Can you work these out from the model? Positions are in its coordinate system, mm. Face numbers are marked on the shaded views. A direction names the side the tool comes from. Coordinates: 2 decimals unless noted, no trailing zeros. Order: outer loops, then holes, each group sorted by start corner. A loop starts at its lowest first (then second) coordinate and runs counter-clockwise, first axis right, second up. Notation, with made-up numbers: (-40, 25.25) -> (16, 25.25) arc R15 cw to (16, 31.25) -> close; hole circle Ø5 at (1.25, 75.25). An arc over 180 degrees is marked (long way). Use a Markdown table: item, result. Add a question column.
1. Suppose I cut it at A-A, the plane x = 0. List the corners of the cut face in (y, z) for me, then the cut area to 3 significant figures.
2. Suppose I cut it at C-C, the plane z = 22. List the corners of the cut face in (x, y) for me, then the cut area to 3 significant figures.
3. Suppose I cut it at B-B, the plane z = 0. List the corners of the cut face in (x, y) for me, then the cut area to 3 significant figures.
4. If I drill on line 1 along Z through (x, y) = (0, -9.4); line 2 along Z through (x, y) = (0, -4.25); line 3 along Y through (x, z) = (-7, 26), over which ranges is the centre line in solid material (lowest first)? Write a range as from..to.
5. Suppose I cut it at D-D, the plane y = -4.75. List the corners of the cut face in (x, z) for me, then the cut area to 3 significant figures.
6. For pin 1 Ø3 at (y, z) = (-3.5, -15.5) entering from -X; pin 2 Ø1.5 at (y, z) = (-3.5, 8.5) entering from +X; pin 3 Ø5 at (x, y) = (-15.5, -1.5) entering from +Z, each with a flat end and sliding along its axis, tell me the tip position at first contact or that it passes through.
7. For the marked faces 1 and 2, which set-ups out of +Z, -Z, +X, -X, +Y, -Y let a thin tool reach every point of the face, with its end or its side?
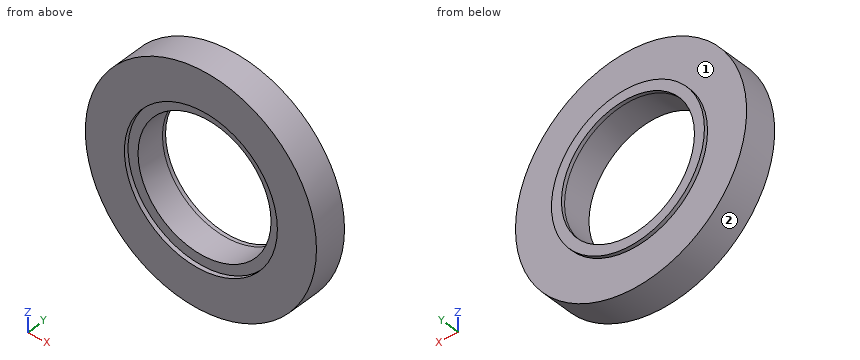
```python
from build123d import *

# Parameters (mm, degrees)
F0_R     = 34.75
F0_R_2   = 20
F1_DEPTH = 10
F2_R     = 23
F2_R_2   = 20
F3_DEPTH = 1.3
F4_R     = 23
F4_R_2   = 20
F5_DEPTH = 1.1


with BuildPart() as f1:
    # F0 (on Front) → F1 (new body)
    with BuildSketch(Plane.XZ):
        Circle(F0_R)
        Circle(F0_R_2, mode=Mode.SUBTRACT)
    extrude(amount=F1_DEPTH)

    # F2 (on face) → F3 (cut)
    with BuildSketch(Plane.XZ.offset(10)):
        Circle(F2_R)
        Circle(F2_R_2, mode=Mode.SUBTRACT)
    extrude(amount=-F3_DEPTH, mode=Mode.SUBTRACT)

    # F4 (on face) → F5 (join)
    with BuildSketch(Plane(origin=(0, 0, 0), x_dir=(-1, 0, 0), z_dir=(0, 1, 0))):
        Circle(F4_R)
        Circle(F4_R_2, mode=Mode.SUBTRACT)
    extrude(amount=F5_DEPTH)


solid = f1.part
```
Worked out:
| question | item | result |
|---|---|---|
| 1 | outline | (-10, -34.75) -> (0, -34.75) -> (0, -23) -> (1.1, -23) -> (1.1, -20) -> (-8.7, -20) -> (-8.7, -23) -> (-10, -23) -> close; (-10, 23) -> (-8.7, 23) -> (-8.7, 20) -> (1.1, 20) -> (1.1, 23) -> (0, 23) -> (0, 34.75) -> (-10, 34.75) -> close |
| 1 | area | 294 mm² |
| 2 | outline | (-26.9, -10) -> (-6.71, -10) -> (-6.71, -8.7) -> (6.71, -8.7) -> (6.71, -10) -> (26.9, -10) -> (26.9, 0) -> (6.71, 0) -> (6.71, 1.1) -> (-6.71, 1.1) -> (-6.71, 0) -> (-26.9, 0) -> close |
| 2 | area | 535 mm² |
| 3 | outline | (-34.75, -10) -> (-23, -10) -> (-23, -8.7) -> (-20, -8.7) -> (-20, 1.1) -> (-23, 1.1) -> (-23, 0) -> (-34.75, 0) -> close; (20, -8.7) -> (23, -8.7) -> (23, -10) -> (34.75, -10) -> (34.75, 0) -> (23, 0) -> (23, 1.1) -> (20, 1.1) -> close |
| 3 | area | 294 mm² |
| 4 | line 1 | z = -34.75..-23, 23..34.75 |
| 4 | line 2 | z = -34.75..-20, 20..34.75 |
| 4 | line 3 | y = -10..0 |
| 5 | outline | circle Ø69.5 at (0, 0); hole circle Ø40 at (0, 0) |
| 5 | area | 2,540 mm² |
| 6 | pin 1 | stops at x = -31.81 |
| 6 | pin 2 | stops at x = 33.87 |
| 6 | pin 3 | stops at z = 32.23 |
| 7 | face 1 | +Y |
| 7 | face 2 | +Y, -Y |
